from build123d import *

# Parameters (mm, degrees)
EXTRUDE_THIN1_DEPTH = 456.40625
FILLET1_R           = 0.889


with BuildPart() as part:
    # Sketch1 → Extrude-Thin1 (new body)
    with BuildSketch(Plane.XY):
        with BuildLine():
            Line((-3.96875, 3.96875), (-3.96875, 6.35))
            Line((-3.96875, 6.35), (0, 6.35))
            Line((0, 6.35), (0, 0))
            Line((0, 0), (-15.875, 0))
            Line((-15.875, 0), (-15.875, 25.4))
            Line((-15.875, 25.4), (-34.925, 25.4))
            Line((-34.925, 25.4), (-34.925, 28.575))
            ThreePointArc((-34.925, 28.575), (-29.089166411, 30.303541744), (-25.13609411, 34.931503458))
            ThreePointArc((-25.13609411, 34.931503458), (-21.402652939, 39.412968218), (-15.875, 41.275))
            Line((-15.875, 41.275), (-15.875, 45.640625))
            Line((-15.875, 45.640625), (0, 45.640625))
            Line((0, 45.640625), (0, 39.290625))
            Line((0, 39.290625), (-3.96875, 39.290625))
            Line((-3.96875, 39.290625), (-3.96875, 43.862625))
            Line((-3.96875, 43.862625), (-3.07975, 43.862625))
            Line((-3.07975, 43.862625), (-3.07975, 40.179625))
            Line((-3.07975, 40.179625), (-0.889, 40.179625))
            Line((-0.889, 40.179625), (-0.889, 44.751625))
            Line((-0.889, 44.751625), (-14.986, 44.751625))
            Line((-14.986, 44.751625), (-14.986, 40.39236674))
            ThreePointArc((-14.986, 40.39236674), (-20.546471616, 38.910847666), (-24.323977473, 34.569857819))
            ThreePointArc((-24.323977473, 34.569857819), (-28.236581443, 29.80735665), (-34.036, 27.720102091))
            Line((-34.036, 27.720102091), (-34.036, 26.289))
            Line((-34.036, 26.289), (-14.986, 26.289))
            Line((-14.986, 26.289), (-14.986, 0.889))
            Line((-14.986, 0.889), (-0.889, 0.889))
            Line((-0.889, 0.889), (-0.889, 5.461))
            Line((-0.889, 5.461), (-3.07975, 5.461))
            Line((-3.07975, 5.461), (-3.07975, 3.96875))
            Line((-3.07975, 3.96875), (-3.96875, 3.96875))
        make_face()
    extrude(amount=-EXTRUDE_THIN1_DEPTH)

    # Fillet1
    fillet1_edges = [part.edges().sort_by_distance(p)[0] for p in [
        (-14.986, 40.39236674, -228.203125),
        (-14.986, 26.289, -228.203125),
        (-3.96875, 6.35, -228.203125),
        (0, 6.35, -228.203125),
        (0, 0, -228.203125),
        (-15.875, 0, -228.203125),
        (-34.925, 25.4, -228.203125),
        (-34.925, 28.575, -228.203125),
        (-15.875, 45.640625, -228.203125),
        (0, 45.640625, -228.203125),
        (0, 39.290625, -228.203125),
        (-3.96875, 39.290625, -228.203125),
    ]]
    fillet(fillet1_edges, radius=FILLET1_R)


solid = part.part
The listing builds one solid part. Answer for the finished solid, in the listing's coordinates (mm). A direction names the side the tool comes from. Give positions to 0.01 mm unless a question says otherwise; leave off trailing zeros. Loops run counter-clockwise (first coordinate to the right, second up) from the corner with the lowest first, then second, coordinate; pieces in that order, holes last. Notation, with made-up numbers: M -14.5,5 L 38.5,5 A11 ccw 38.5,14 Z; hole C 59,79.25 d7. An arc over 180 degrees is marked long. Answer as CSV lines item,"result".
Item 1: The part is cut by section A-A (y = 12.5). Give the vertices of the cut face in (x, z) (3 decimals).
Values follow:
outline,"M -15.875,-456.406 L -14.986,-456.406 L -14.986,0 L -15.875,0 Z"
Item 2: Which of the six approach directions +Z, -Z, +X, -X, +Y, -Y give full straight-line access (tool end or side, diameter ignored) to faces 1 (the flat face through (-19, 40, 0)), 2 (the flat face through (-14.986, 13, -225)), 3 (the flat face through (-15.875, 13, -225)), 4 (the flat face through (-25, 26.289, -225)), 5 (the flat face through (-8, 0, -225))?
Values follow:
face 1,"+Z, +X, -X, +Y, -Y"
face 2,"+Z, -Z"
face 3,"+Z, -Z, -X, -Y"
face 4,"+Z, -Z, +X"
face 5,"+Z, -Z, +X, -X, -Y"
Item 3: The mould has two halves that part along Y. Classify faces 6 (the flat face through (-8, 45.641, -225)), 7 (the flat face through (-19, 40, -456.406)), 8 (the flat face through (-8, 44.752, -225)): released by +Y, released by -Y, zero draft, split by the parting line, or undercut.
Values follow:
face 6,"released by +Y"
face 7,"zero draft"
face 8,"undercut"
Item 4: Straight lines are drawn through the part: line 1 along X through (y, z) = (41.5, -127) (3 decimals); line 2 along Y through (x, z) = (-12, -210.5); line 3 along Y through (x, z) = (-3.5, -205.5). For each, find the intervals that lie inside material, in ascending order. Write a range as [from, to].
Values follow:
line 1,"x = [-15.875, -14.986], [-3.969, -3.08], [-0.889, 0]"
line 2,"y = [0, 0.89], [44.75, 45.64]"
line 3,"y = [0, 0.89], [3.97, 6.24], [39.4, 43.86], [44.75, 45.64]"
Item 5: Given pin 1 Ø3 at (y, z) = (41, -238.5) entering from -X; pin 2 Ø7.5 at (y, z) = (9.5, -288.5) entering from +X; pin 3 Ø20 at (x, z) = (-25.5, -302.5) entering from +Y; pin 4 Ø6 at (x, y) = (-11.5, 38) entering from -Z, each flat-ended and moving along its own axis, determine where each tip first touches the part or whether it passes through.
Values follow:
pin 1,"stops at x = -21.27"
pin 2,"stops at x = -0.05"
pin 3,"stops at y = 45.48"
pin 4,"passes through"
